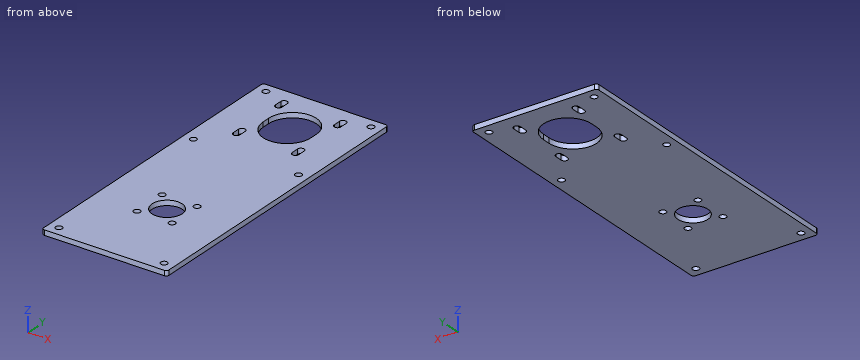
from build123d import *

# Parameters (mm, degrees)
SKETCH1_R           = 2.625
SKETCH1_R_2         = 12
BOSS_EXTRUDE1_DEPTH = 4


with BuildPart() as part:
    # Sketch1 → Boss-Extrude1 (new body)
    with BuildSketch(Plane.XY.offset(4)):
        with BuildLine():
            Line((-48, -123.5), (48, -123.5))
            ThreePointArc((48, -123.5), (49.414213562, -122.914213562), (50, -121.5))
            Line((50, -121.5), (50, 121.5))
            ThreePointArc((50, 121.5), (49.414213562, 122.914213562), (48, 123.5))
            Line((48, 123.5), (-48, 123.5))
            ThreePointArc((-48, 123.5), (-49.414213562, 122.914213562), (-50, 121.5))
            Line((-50, 121.5), (-50, -121.5))
            ThreePointArc((-50, -121.5), (-49.414213562, -122.914213562), (-48, -123.5))
        make_face()
        with Locations(Location((14, -67.5, 0), (0, 0, 180))):
            Circle(SKETCH1_R, mode=Mode.SUBTRACT)
        with Locations(Location((-14, -67.5, 0), (0, 0, 180))):
            Circle(SKETCH1_R, mode=Mode.SUBTRACT)
        with Locations(Location((14, -39.5, 0), (0, 0, 180))):
            Circle(SKETCH1_R, mode=Mode.SUBTRACT)
        with Locations(Location((42, 115.5, 0), (0, 0, 180))):
            Circle(SKETCH1_R, mode=Mode.SUBTRACT)
        with Locations(Location((0, -53.5, 0), (0, 0, 180))):
            Circle(SKETCH1_R_2, mode=Mode.SUBTRACT)
        with Locations(Location((-42, 34.5, 0), (0, 0, 180))):
            Circle(SKETCH1_R, mode=Mode.SUBTRACT)
        with Locations(Location((-42, -115.5, 0), (0, 0, 180))):
            Circle(SKETCH1_R, mode=Mode.SUBTRACT)
        with Locations(Location((-14, -39.5, 0), (0, 0, 180))):
            Circle(SKETCH1_R, mode=Mode.SUBTRACT)
        with Locations(Location((42, 34.5, 0), (0, 0, 180))):
            Circle(SKETCH1_R, mode=Mode.SUBTRACT)
        with Locations(Location((42, -115.5, 0), (0, 0, 180))):
            Circle(SKETCH1_R, mode=Mode.SUBTRACT)
        with Locations(Location((-42, 115.5, 0), (0, 0, 180))):
            Circle(SKETCH1_R, mode=Mode.SUBTRACT)
        with BuildLine():
            Line((-26.13, 57), (-26.13, 63))
            ThreePointArc((-26.13, 63), (-23.5, 65.63), (-20.87, 63))
            Line((-20.87, 63), (-20.87, 57))
            ThreePointArc((-20.87, 57), (-23.5, 54.37), (-26.13, 57))
        make_face(mode=Mode.SUBTRACT)
        with BuildLine():
            Line((20.87, 104), (20.87, 110))
            ThreePointArc((20.87, 110), (23.5, 112.63), (26.13, 110))
            Line((26.13, 110), (26.13, 104))
            ThreePointArc((26.13, 104), (23.5, 101.37), (20.87, 104))
        make_face(mode=Mode.SUBTRACT)
        with BuildLine():
            Line((-19.05, 80.5), (-19.05, 86.5))
            ThreePointArc((-19.05, 86.5), (0, 105.55), (19.05, 86.5))
            Line((19.05, 86.5), (19.05, 80.5))
            ThreePointArc((19.05, 80.5), (0, 61.45), (-19.05, 80.5))
        make_face(mode=Mode.SUBTRACT)
        with BuildLine():
            Line((26.13, 63), (26.13, 57))
            ThreePointArc((26.13, 57), (23.5, 54.37), (20.87, 57))
            Line((20.87, 57), (20.87, 63))
            ThreePointArc((20.87, 63), (23.5, 65.63), (26.13, 63))
        make_face(mode=Mode.SUBTRACT)
        with BuildLine():
            Line((-20.87, 110), (-20.87, 104))
            ThreePointArc((-20.87, 104), (-23.5, 101.37), (-26.13, 104))
            Line((-26.13, 104), (-26.13, 110))
            ThreePointArc((-26.13, 110), (-23.5, 112.63), (-20.87, 110))
        make_face(mode=Mode.SUBTRACT)
    extrude(amount=-BOSS_EXTRUDE1_DEPTH)


solid = part.part
Geometry: final body of the model. Coordinates: model frame, mm. Coordinates: 2 decimals unless noted, no trailing zeros. Loops run counter-clockwise (first coordinate to the right, second up) from the corner with the lowest first, then second, coordinate; pieces in that order, holes last. Notation, with made-up numbers: (-3, 27) - (24, 27) arc R13 ccw to (24, 46) - close; hole circle Ø2 at (37, 6.25). An arc over 180 degrees is marked (long way). Put each result on its own line as item: value. Start each with the question number.
Q1. Cut plane B-B, the plane y = -53.5. Return loops of the section in (x, z).
Q2. Cut plane A-A, the plane y = 115.5. Return loops of the section in (x, z) (3 decimals).
Q3. Pin query (flat end, axial travel): pin 1 Ø2 at (x, y) = (3, -87) entering from -Z; pin 2 Ø4.5 at (x, y) = (14, -67.5) entering from -Z. Return the tip coordinate at first contact, or that it passes through.
Q4. Line query: line 1 (X direction, y = 108, z = 3.4); line 2 (Y direction, x = 42, z = 2.95) (3 decimals); line 3 (X direction, y = 34.5, z = 1.4) (3 decimals). Output: solid intervals per line, ascending.
Q5. Cut plane C-C, the plane z = 2.15. Give the number of separate pieces and of enclosed holes in the cut face, and give its area (3 significant figures).
Filled sheet:
1. outline: (-50, 0) - (-12, 0) - (-12, 4) - (-50, 4) - close; (12, 0) - (50, 0) - (50, 4) - (12, 4) - close
2. outline: (-50, 0) - (-44.625, 0) - (-44.625, 4) - (-50, 4) - close; (-39.375, 0) - (39.375, 0) - (39.375, 4) - (-39.375, 4) - close; (44.625, 0) - (50, 0) - (50, 4) - (44.625, 4) - close
3. pin 1: z = 0
3. pin 2: through
4. line 1: -50 to -26.13, -20.87 to 20.87, 26.13 to 50
4. line 2: -123.5 to -118.125, -112.875 to 31.875, 37.125 to 112.875, 118.125 to 123.5
4. line 3: -50 to -44.625, -39.375 to 39.375, 44.625 to 50
5. separate pieces: 1
5. enclosed holes: 16
5. area: 22,400 mm²
